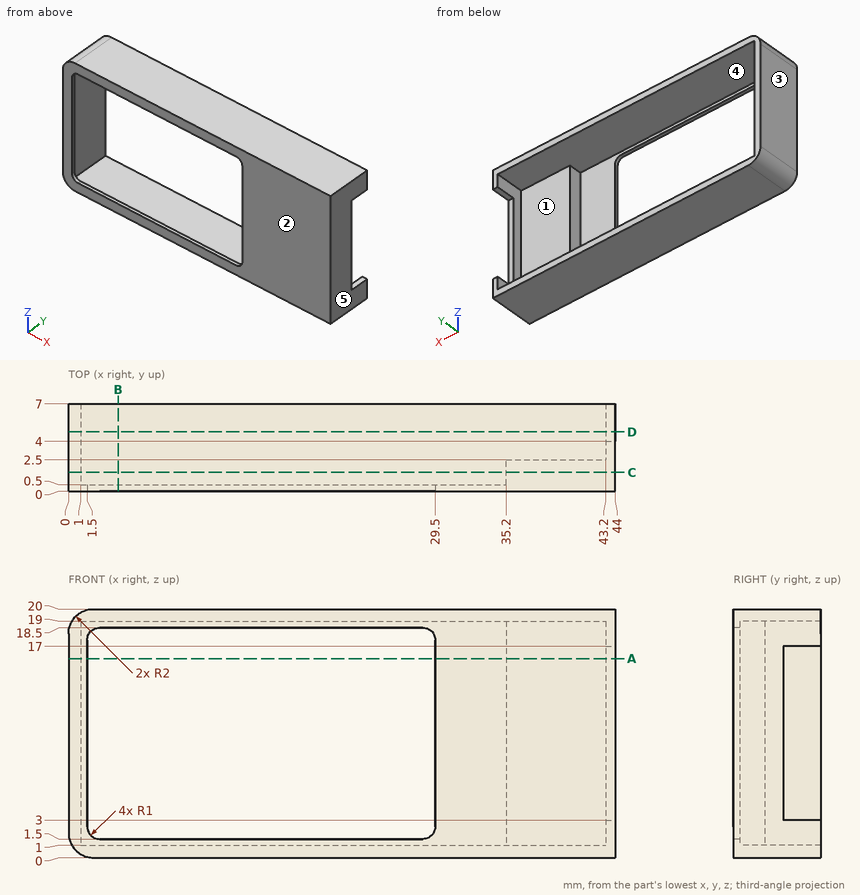
Study the drawing (mm; zero at the part's minimum x, y, z) and answer. A direction names the side the tool comes from. Give positions to 0.01 mm unless a question says otherwise; leave off trailing zeros. Write each loop counter-clockwise with the first axis right and the second up, starting at its lowest first coordinate (ties: lowest second). Pieces come first, ordered by that corner, then holes. Notation, with made-up numbers: (31, 4) - (57, 4) arc R17 ccw to (57, 15) - close; hole circle Ø11 at (-24.5, -31). An arc over 180 degrees is marked (long way). Use a Markdown table: item, result.
1. Section C-C on y = 1.5 is taken. Write down the section's boundary in (x, z), plus the area to 3 significant figures.
Values follow:
| item | result |
|---|---|
| outline | (0, 2) arc R2 ccw to (2, 0) - (44, 0) - (44, 20) - (2, 20) arc R2 ccw to (0, 18) - close; hole (1, 1) - (35.2, 1) - (35.2, 19) - (1, 19) - close |
| area | 263 mm² |
2. A tool of negligible diameter and unlimited length cuts with its end or side. For the marked faces 1 and 2, from which of +Z, -Z, +X, -X, +Y, -Y can it reach the whole face along a straight path? Write none if from no direction.
Values follow:
| item | result |
|---|---|
| face 1 | +Y |
| face 2 | +Z, -Z, +X, -X, -Y |
3. Section A-A on z = 16 is taken. Write down the section's boundary in (x, y).
Values follow:
| item | result |
|---|---|
| outline | (0, 0) - (1.5, 0) - (1.5, 0.5) - (1, 0.5) - (1, 7) - (0, 7) - close; (29.5, 0) - (44, 0) - (44, 4) - (43.2, 4) - (43.2, 2.5) - (35.2, 2.5) - (35.2, 0.5) - (29.5, 0.5) - close |
4. This flat-tipped pin is pushed along its axis until it touches: P1, Ø9, axis at x = 40.5, z = 9, coming from the +Y side. Where does it stop, or does it pass through?
Values follow:
| item | result |
|---|---|
| P1 | stops at y = 4 |
5. For a pull along X with two mould halves and no side action, classify the marked faces 3, 4 and 5 as released by +X, released by -X, zero draft, split by the parting line, or undercut.
Values follow:
| item | result |
|---|---|
| face 3 | released by -X |
| face 4 | undercut |
| face 5 | released by +X |
6. Section D-D on y = 4.75 is taken. Write down the section's boundary in (x, z).
Values follow:
| item | result |
|---|---|
| outline | (0, 2) arc R2 ccw to (2, 0) - (44, 0) - (44, 3) - (43.2, 3) - (43.2, 1) - (1, 1) - (1, 19) - (43.2, 19) - (43.2, 17) - (44, 17) - (44, 20) - (2, 20) arc R2 ccw to (0, 18) - close |
7. Section B-B on x = 4 is taken. Write down the section's boundary in (y, z), plus the area to 3 significant figures.
Values follow:
| item | result |
|---|---|
| outline | (0, 0) - (7, 0) - (7, 1) - (0.5, 1) - (0.5, 1.5) - (0, 1.5) - close; (0, 18.5) - (0.5, 18.5) - (0.5, 19) - (7, 19) - (7, 20) - (0, 20) - close |
| area | 14.5 mm² |
8. Find the intervals of material crossed by probe 1 along Z at (x, y) = (17.5, 5.25); probe 2 along X at (y, z) = (1.5, 3); probe 3 along X at (y, z) = (5, 13), in increasing order. Write a range as from..to.
Values follow:
| item | result |
|---|---|
| probe 1 | z = 0..1, 19..20 |
| probe 2 | x = 0..1, 35.2..44 |
| probe 3 | x = 0..1 |
